Geometry: final body of the model. Coordinates: model frame, mm. A direction names the side the tool comes from. Coordinates: 2 decimals unless noted, no trailing zeros. Loops run counter-clockwise (first coordinate to the right, second up) from the corner with the lowest first, then second, coordinate; pieces in that order, holes last. Notation, with made-up numbers: (30.5, 87) - (47.5, 87) arc R10 cw to (47.5, 102) - close; hole circle Ø7 at (46.25, -19). An arc over 180 degrees is marked (long way). Return JSON: item names as keys, results as strings.
from build123d import *

# Parameters (mm, degrees)
EXTRUDE_THIN1_DEPTH = 635
FILLET1_R           = 1.143


with BuildPart() as part:
    # Sketch1 → Extrude-Thin1 (new body)
    with BuildSketch(Plane.XY):
        with BuildLine():
            Line((0, 0), (-23.8125, 0))
            Line((-23.8125, 0), (-23.8125, 3.96875))
            ThreePointArc((-23.8125, 3.96875), (-30.547692, 6.758558), (-33.3375, 13.49375))
            Line((-33.3375, 13.49375), (-36.5125, 13.49375))
            Line((-36.5125, 13.49375), (-36.5125, 33.437109))
            ThreePointArc((-36.5125, 33.437109), (-39.6875, 41.83737), (-47.625, 46.0375))
            Line((-47.625, 46.0375), (-47.625, 63.5))
            Line((-47.625, 63.5), (-7.9375, 63.5))
            Line((-7.9375, 63.5), (-7.9375, 62.357))
            Line((-7.9375, 62.357), (-46.482, 62.357))
            Line((-46.482, 62.357), (-46.482, 47.008145))
            ThreePointArc((-46.482, 47.008145), (-38.502062, 42.207239), (-35.3695, 33.437109))
            Line((-35.3695, 33.437109), (-35.3695, 14.63675))
            Line((-35.3695, 14.63675), (-32.116202, 14.63675))
            ThreePointArc((-32.116202, 14.63675), (-29.739469, 7.566781), (-22.6695, 5.190048))
            Line((-22.6695, 5.190048), (-22.6695, 1.143))
            Line((-22.6695, 1.143), (0, 1.143))
            Line((0, 1.143), (0, 0))
        make_face()
    extrude(amount=-EXTRUDE_THIN1_DEPTH)

    # Fillet1
    fillet1_edges = [part.edges().sort_by_distance(p)[0] for p in [
        (-32.116202, 14.63675, -317.5),
        (-22.6695, 5.190048, -317.5),
        (-23.8125, 0, -317.5),
        (-36.5125, 13.49375, -317.5),
        (-47.625, 46.0375, -317.5),
        (-47.625, 63.5, -317.5),
    ]]
    fillet(fillet1_edges, radius=FILLET1_R)


solid = part.part
Item 1: Section query A-A, the plane x = -15. Return loops of the section in (y, z), and give its area (3 significant figures).
Worked out:
{"outline": "(0, -635) - (1.14, -635) - (1.14, 0) - (0, 0) - close; (62.36, -635) - (63.5, -635) - (63.5, 0) - (62.36, 0) - close", "area": "1,450 mm^2"}
Item 2: Section query C-C, the plane y = 24. Return loops of the section in (x, z).
Worked out:
{"outline": "(-36.51, -635) - (-35.37, -635) - (-35.37, 0) - (-36.51, 0) - close"}
Item 3: Reachability of faces 1 (the face through (-11, 1.143, -313)), 2 (the face through (-36.512, 24, -313)), 3 (the face through (-11, 0, -313)) from +Z, -Z, +X, -X, +Y, -Y: full face, straight path, thin tool, end or side. Return the list, or none.
Worked out:
{"face 1": "+Z, -Z, +X", "face 2": "+Z, -Z, -X, -Y", "face 3": "+Z, -Z, +X, -X, -Y"}
Item 4: Mould query, pull axis Y, two halves, no side actions, for faces 4 (the face through (-35.37, 24, -313)), 5 (the face through (-27, 63.5, -313)), 6 (the face through (-41, 44, 0)). Classes: +Y half, -Y half, draft (parallel to the pull), parting line (faces both ways), or undercut.
Worked out:
{"face 4": "undercut", "face 5": "+Y half", "face 6": "draft"}
Item 5: First-contact query: pin 1 Ø2 at (y, z) = (11, -149) entering from -X; pin 2 Ø1.4 at (y, z) = (2.5, -176) entering from -X; pin 3 Ø1.4 at (y, z) = (2.5, -388) entering from +X. Flat tips, straight axial feed; report the tip coordinate or a pass-through.
Worked out:
{"pin 1": "x = -33.22", "pin 2": "x = -23.81", "pin 3": "x = -22.67"}
Item 6: Ray query, probe 1 along Y at (x, z) = (-18, -78); probe 2 along X at (y, z) = (3.5, -102.5); probe 3 along Y at (x, z) = (-24.5, -524). Return the intervals inside material, ascending. Write a range as from..to.
Worked out:
{"probe 1": "0..1.14, 62.36..63.5", "probe 2": "-23.81..-22.67", "probe 3": "3.99..5.14, 62.36..63.5"}
